The model under review builds one solid part; all positions refer to its coordinate system, in mm. A direction names the side the tool comes from. Coordinates: 2 decimals unless noted, no trailing zeros. Answer in a Markdown table with one row per item.
```python
from build123d import *

# Parameters (mm, degrees)
CROQUIS1_W              = 20
CROQUIS1_H              = 132
SALIENTE_EXTRUIR1_DEPTH = 7
CROQUIS2_RX             = 3.2
CROQUIS2_RY             = 2.375
CORTAR_EXTRUIR1_DEPTH   = 0.2


with BuildPart() as part:
    # Croquis1 → Saliente-Extruir1 (new body)
    with BuildSketch(Plane(origin=(0, 0, 0), x_dir=(1, 0, 0), z_dir=(0, 1, 0))):
        Rectangle(CROQUIS1_W, CROQUIS1_H)
    extrude(amount=SALIENTE_EXTRUIR1_DEPTH)

    # Croquis2 → Cortar-Extruir1 (cut)
    with BuildSketch(Plane(origin=(0, 7, 0), x_dir=(1, 0, 0), z_dir=(0, 1, 0))):
        with Locations(Location((0.008026014, -59), (0, 0, -125.538109025))):
            Ellipse(CROQUIS2_RX, CROQUIS2_RY)
        with Locations(Location((0.000308673, 1.309257057), (0, 0, 54.461890975))):
            Ellipse(CROQUIS2_RX, CROQUIS2_RY)
        with Locations(Location((0.000308673, -1.309627052), (0, 0, -54.461890975))):
            Ellipse(CROQUIS2_RX, CROQUIS2_RY)
        with Locations(Location((0.008026014, 58.999630006), (0, 0, -54.461890975))):
            Ellipse(CROQUIS2_RX, CROQUIS2_RY)
    extrude(amount=-CORTAR_EXTRUIR1_DEPTH, mode=Mode.SUBTRACT)


solid = part.part
```
Item 1: Clearance check with flat-ended pins moving along their axes: pin 1 Ø4 at (x, z) = (-7.5, -41) entering from -Y; pin 2 Ø1.6 at (x, z) = (0.5, -58.5) entering from +Y. State where each tip first meets the part, or that it passes through.
Check values:
| item | result |
|---|---|
| pin 1 | y = 0 |
| pin 2 | y = 6.8 |
Item 2: Tool access review of faces 4 (the face through (-10, 3, 1)), 5 (the face through (0, 6.8, 59)): name each direction out of +Z, -Z, +X, -X, +Y, -Y from which nothing blocks a thin tool from reaching the whole face with its end or side.
Check values:
| item | result |
|---|---|
| face 4 | +Z, -Z, -X, +Y, -Y |
| face 5 | +Y |
Item 3: To check wall thickness, follow line 1 (Y direction, x = -0.5, z = 0). State the ranges of the line that lie inside material, in increasing order. Write a range as from..to.
Check values:
| item | result |
|---|---|
| line 1 | 0..6.8 |
Item 4: Mouldability with a two-part tool opening along Z and no side actions: class faces 1 (the face through (0, 6.8, 0)), 2 (the face through (0, 3, -66)), 3 (the face through (0, 0, -1)) as +Z half, -Z half, draft (parallel to the pull), parting line (faces both ways), or undercut.
Check values:
| item | result |
|---|---|
| face 1 | undercut |
| face 2 | -Z half |
| face 3 | draft |
